```python
from build123d import *

# Parameters (mm, degrees)
SKETCH_1_R          = 2.25
SKETCH_1_R_2        = 1.75
EXTRUDE_1_DEPTH     = 10
SKETCH_3_W          = 7
SKETCH_3_H          = 7
CUT_EXTRUDE_1_DEPTH = 276.22717889
EXTRUDE_2_DEPTH     = 4
SKETCH_7_R          = 1
CUT_EXTRUDE_2_DEPTH = 2
SKETCH_8_W          = 6.516904704
SKETCH_8_H          = 4
CUT_EXTRUDE_3_DEPTH = 3
SKETCH_9_W          = 1.9
SKETCH_9_H          = 5
EXTRUDE_3_DEPTH     = 24.5
SKETCH_10_W         = 5
SKETCH_10_H         = 5
EXTRUDE_4_DEPTH     = 14.2
EXTRUDE_9_DEPTH     = 4
SKETCH_12_R         = 1
CUT_EXTRUDE_4_DEPTH = 3
EXTRUDE_10_DEPTH    = 11.25
SKETCH_14_W         = 18.9
SKETCH_14_H         = 20.745864208
EXTRUDE_13_DEPTH    = 2
SKETCH_15_W         = 12
SKETCH_15_H         = 0.3
CUT_EXTRUDE_5_DEPTH = 272.22739998
SKETCH_16_W         = 16
SKETCH_16_H         = 10
EXTRUDE_14_DEPTH    = 10
FILLET_1_R          = 4
SKETCH_17_R         = 4.04
CUT_EXTRUDE_7_DEPTH = 10
SKETCH_20_R         = 7
SKETCH_20_R_2       = 4.04
EXTRUDE_15_DEPTH    = 10
FILLET_3_R          = 3.5
SKETCH_21_R         = 4.15
CUT_EXTRUDE_8_DEPTH = 10


with BuildPart() as part:
    # 草图1 → 凸台-拉伸1 (new body)
    with BuildSketch(Plane.XY):
        with BuildLine():
            Line((265, 5), (-5, 5))
            Line((-5, 5), (-5, -5))
            Line((-5, -5), (265, -5))
            ThreePointArc((265, -5), (270, 0), (265, 5))
        make_face()
        Circle(SKETCH_1_R, mode=Mode.SUBTRACT)
        with Locations((165, 0)):
            Circle(SKETCH_1_R_2, mode=Mode.SUBTRACT)
        with Locations((265, 0)):
            Circle(SKETCH_1_R_2, mode=Mode.SUBTRACT)
    extrude(amount=-EXTRUDE_1_DEPTH)

    # 草图3 → 切除-拉伸1 (cut, through all)
    with BuildSketch(Plane.ZY.offset(5)):
        with Locations((-5, 0)):
            Rectangle(SKETCH_3_W, SKETCH_3_H)
    extrude(amount=-CUT_EXTRUDE_1_DEPTH, mode=Mode.SUBTRACT)

    # 草图5 → 凸台-拉伸2 (add)
    with BuildSketch(Plane(origin=(0, 0, -10), x_dir=(-1, 0, 0), z_dir=(0, 0, -1))):
        Polygon((5, 5), (18.9, 5), (18.9, 0), (0, 0), (0, 5), align=None)
    extrude(amount=EXTRUDE_2_DEPTH)

    # 草图7 → 切除-拉伸2 (cut)
    with BuildSketch(Plane(origin=(0, 5, 0), x_dir=(1, 0, 0), z_dir=(0, 1, 0))):
        with Locations(Location((-10.95, 11.9, 0), (0, 0, 180))):
            Circle(SKETCH_7_R)
    extrude(amount=-CUT_EXTRUDE_2_DEPTH, mode=Mode.SUBTRACT)

    # 草图8 → 切除-拉伸3 (cut)
    with BuildSketch(Plane.XZ):
        with Locations((-10.951938586, -12)):
            Rectangle(SKETCH_8_W, SKETCH_8_H)
    extrude(amount=-CUT_EXTRUDE_3_DEPTH, mode=Mode.SUBTRACT)

    # 草图9 → 凸台-拉伸3 (add)
    with BuildSketch(Plane.XY.offset(-10)):
        with Locations((-17.95, 2.5)):
            Rectangle(SKETCH_9_W, SKETCH_9_H)
    extrude(amount=EXTRUDE_3_DEPTH)

    # 草图10 → 凸台-拉伸4 (add)
    with BuildSketch(Plane.XY):
        with Locations((-2.5, 2.5)):
            Rectangle(SKETCH_10_W, SKETCH_10_H)
    extrude(amount=EXTRUDE_4_DEPTH)

    # 草图11 → 凸台-拉伸9 (add)
    with BuildSketch(Plane.XY.offset(14.2)):
        Polygon((0, 0), (-7.693486234, 0), (-7.693486234, 3), (-14.210390938, 3), (-14.210390938, 0), (-18.9, 0), (-18.9, 5), (0, 5), align=None)
    extrude(amount=EXTRUDE_9_DEPTH)

    # 草图12 → 切除-拉伸4 (cut)
    with BuildSketch(Plane(origin=(0, 5, 0), x_dir=(1, 0, 0), z_dir=(0, 1, 0))):
        with Locations(Location((-10.95, -15.9, 0), (0, 0, 180))):
            Circle(SKETCH_12_R)
    extrude(amount=-CUT_EXTRUDE_4_DEPTH, mode=Mode.SUBTRACT)

    # 草图13 → 凸台-拉伸10 (add)
    with BuildSketch(Plane.XZ):
        Polygon((-14.210390938, -14), (-14.210390938, -10), (-17, -10), (-17, 14.2), (-14.210390938, 14.2), (-14.210390938, 18.2), (-18.9, 18.2), (-18.9, -14), align=None)
        Polygon((-7.693486234, -14), (0, -14), (0, -10), (0, 18.2), (-7.693486234, 18.2), (-7.693486234, 14.2), (-5, 14.2), (-5, -10), (-7.693486234, -10), align=None)
    extrude(amount=EXTRUDE_10_DEPTH)

    # 草图14 → 凸台-拉伸13 (add)
    with BuildSketch(Plane(origin=(0, -11.25, 0), x_dir=(-1, 0, 0), z_dir=(0, -1, 0))):
        with Locations((9.45, -1.594289746)):
            Rectangle(SKETCH_14_W, SKETCH_14_H)
    extrude(amount=EXTRUDE_13_DEPTH)

    # 草图15 → 切除-拉伸5 (cut, through all)
    with BuildSketch(Plane(origin=(0, 5, 0), x_dir=(1, 0, 0), z_dir=(0, 1, 0))):
        with Locations((-11, 10.15)):
            Rectangle(SKETCH_15_W, SKETCH_15_H)
    extrude(amount=-CUT_EXTRUDE_5_DEPTH, mode=Mode.SUBTRACT)

    # 草图16 → 凸台-拉伸14 (add)
    with BuildSketch(Plane.XY):
        with Locations((165, 0)):
            Rectangle(SKETCH_16_W, SKETCH_16_H)
        with Locations((265, 0)):
            Rectangle(SKETCH_16_W, SKETCH_16_H)
    extrude(amount=-EXTRUDE_14_DEPTH)

    # 圆角1
    fillet_1_edges = [part.edges().sort_by_distance(p)[0] for p in [
        (273, -5, -5),
        (273, 5, -5),
    ]]
    fillet(fillet_1_edges, radius=FILLET_1_R)

    # 草图17 → 切除-拉伸7 (cut)
    with BuildSketch(Plane.XY):
        with Locations((165, 0)):
            Circle(SKETCH_17_R)
        with Locations((265, 0)):
            Circle(SKETCH_17_R)
    extrude(amount=-CUT_EXTRUDE_7_DEPTH, mode=Mode.SUBTRACT)

    # 草图20 → 凸台-拉伸15 (add)
    # profile 1 of 2: a face of its own
    with BuildSketch(Plane.XY):
        with Locations((165, 0)):
            Circle(SKETCH_20_R)
        with Locations((165, 0)):
            Circle(SKETCH_20_R_2, mode=Mode.SUBTRACT)
    # profile 2 of 2: a face of its own
    with BuildSketch(Plane.XY):
        with Locations((265, 0)):
            Circle(SKETCH_20_R)
        with Locations((265, 0)):
            Circle(SKETCH_20_R_2, mode=Mode.SUBTRACT)
    extrude(amount=-EXTRUDE_15_DEPTH)

    # 圆角3
    # the kernel refuses this fillet: 3.5 mm, written as the material it adds along each edge
    with BuildSketch(Plane(origin=(-5, 3.5, -8.5), x_dir=(0, -1, 0), z_dir=(1, 0, 0))) as fillet_3_piece_1_section:
        with BuildLine():
            CenterArc((FILLET_3_R, -FILLET_3_R), FILLET_3_R, 90, 90)
            Line((0, -FILLET_3_R), (0, 0))
            Line((0, 0), (FILLET_3_R, 0))
        make_face()
    fillet_3_piece_1 = extrude(amount=162, mode=Mode.PRIVATE)
    fillet_3_piece_1 = fillet_3_piece_1 - Plane(origin=(0, 0, -7.682274374), x_dir=(1, 0, 0), z_dir=(0, 0, 1)) * Cylinder(2.25, 339, mode=Mode.PRIVATE)
    add(fillet_3_piece_1)
    with BuildSketch(Plane(origin=(-5, 3.5, -1.5), x_dir=(0, -1, 0), z_dir=(1, 0, 0))) as fillet_3_piece_2_section:
        with BuildLine():
            CenterArc((FILLET_3_R, FILLET_3_R), FILLET_3_R, 180, 90)
            Line((0, FILLET_3_R), (0, 0))
            Line((0, 0), (FILLET_3_R, 0))
        make_face()
    fillet_3_piece_2 = extrude(amount=162, mode=Mode.PRIVATE)
    fillet_3_piece_2 = fillet_3_piece_2 - Plane(origin=(0, 0, -2.317725626), x_dir=(1, 0, 0), z_dir=(0, 0, 1)) * Cylinder(2.25, 339, mode=Mode.PRIVATE)
    add(fillet_3_piece_2)

    # 草图21 → 切除-拉伸8 (cut)
    with BuildSketch(Plane.XY):
        with Locations((165, 0)):
            Circle(SKETCH_21_R)
        with Locations((265, 0)):
            Circle(SKETCH_21_R)
    extrude(amount=-CUT_EXTRUDE_8_DEPTH, mode=Mode.SUBTRACT)


solid = part.part
```
Check sheet for the modelled part. Datum: model origin and axes. Units: mm. A direction names the side the tool comes from. Round coordinates to 2 decimals unless told otherwise and drop trailing zeros. Loops run counter-clockwise (first coordinate to the right, second up) from the corner with the lowest first, then second, coordinate; pieces in that order, holes last. Notation, with made-up numbers: (34, -9.5) - (90, -9.5) arc R37 ccw to (90, 28.5) - close; hole circle Ø7 at (86, 28.5). An arc over 180 degrees is marked (long way). Answer as a JSON object with one key per item and string values. Group by question number.
Q1. Mould release check, pull along Z, two halves, no side actions. Record for faces 6 (the face through (257, 0, -5)), 7 (the face through (265, 7, -5)): released by +Z, released by -Z, zero draft, split by the parting line, or undercut.
Q2. Gauge pin test, flat ends, axial feed: P1, Ø3, axis at x = 70, y = -7.5, coming from the +Z side; P2, Ø5, axis at x = 100, z = 0.5, coming from the +Y side; P3, Ø2, axis at x = 199, y = -1.5, coming from the -Z side; P4, Ø3, axis at x = -3.5, z = 15.5, coming from the -Y side. Record the tip position at first contact, or that the pin passes through.
Q3. Sectioned sample at B-B, the plane x = 165. Enter the section's corners in (y, z).
Q4. Sectioned sample at A-A, the plane x = 247.5. Enter the section's corners in (y, z).
Q5. Set-up check for faces 1 (the face through (214, -5, -5)), 2 (the face through (214, 0, -1.5)), 3 (the face through (-11, -11.25, 1)), 4 (the face through (-15, -3, -10.3)), 5 (the face through (-18.9, -4, 2)): record each of +Z, -Z, +X, -X, +Y, -Y from which the full face is reachable in a straight line by a thin tool's end or side.
Q6. Scan lines: line 1 along X through (y, z) = (2, 11); line 2 along Y through (x, z) = (191, -5); line 3 along Z through (x, y) = (152, -2). Record each from-to range of solid material in increasing order. Write a range as [from, to].
Solution:
{
 "1": {"face 6": "undercut", "face 7": "zero draft"},
 "2": {"P1": "passes through", "P2": "stops at y = 5", "P3": "stops at z = -10", "P4": "stops at y = -11.25"},
 "3": {"outline": "(-7, -10) - (-4.15, -10) - (-4.15, 0) - (-7, 0) - close; (4.15, -10) - (7, -10) - (7, 0) - (4.15, 0) - close"},
 "4": {"outline": "(-5, -10) - (5, -10) - (5, 0) - (-5, 0) - close; hole (-3.5, -8.5) - (3.5, -8.5) - (3.5, -1.5) - (-3.5, -1.5) - close"},
 "5": {"face 1": "+Z, -Z, -Y", "face 2": "none", "face 3": "+Y", "face 4": "+Y, -Y", "face 5": "+Z, -Z, -X, +Y, -Y"},
 "6": {"line 1": "x = [-18.9, -17], [-5, 0]", "line 2": "y = [-5, -3.5], [3.5, 5]", "line 3": "z = [-10, -8.5], [-1.5, 0]"}
}
